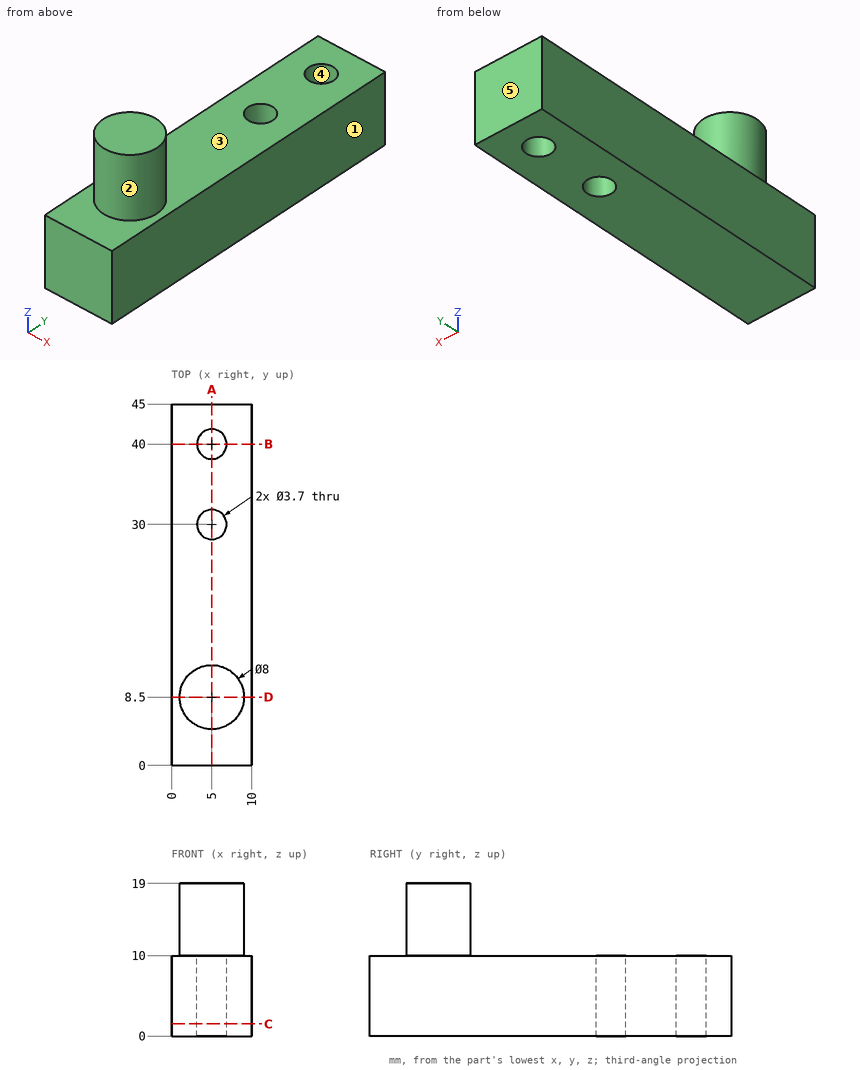
Job drawing, mm, ordinate dimensions from the low corner. One solid piece. A direction names the side the tool comes from. Give positions to 0.01 mm unless a question says otherwise; leave off trailing zeros. Loops run counter-clockwise (first coordinate to the right, second up) from the corner with the lowest first, then second, coordinate; pieces in that order, holes last. Notation, with made-up numbers: (-8, 26.25) -> (17, 26.25) arc R26 cw to (17, 40.25) -> close; hole circle Ø3 at (55.5, 30). An arc over 180 degrees is marked (long way). Use a Markdown table: item, result. Add a question column.
(1) Slice it at C-C on z = 1.5. List the corners of the cut face in (x, y).
(2) Drop a flat-ended pin along its axis: pin 1 Ø3 at (x, y) = (5.5, 24) entering from +Z. Give the stop position or say it passes through.
(3) Tool access for the marked faces 1 and 2: list every direction of +Z, -Z, +X, -X, +Y, -Y with a clear straight run to the whole face (end or side of a thin tool).
(4) Slice it at B-B on y = 40. List the corners of the cut face in (x, z), and give its area (3 significant figures).
(5) Slice it at A-A on x = 5. List the corners of the cut face in (y, z).
(6) Wall check: line 1 along Y through (x, z) = (5, 6.25); line 2 along Z through (x, y) = (9, 5.5); line 3 along X through (y, z) = (39, 8.25). Give the ranges that are in metal, low to high.
(7) Mould opens along Y. For the marked faces 3, 4 and 5 say: +Y half, -Y half, draft (parallel to the pull), parting line (faces both ways), or undercut.
(8) Slice it at D-D on y = 8.5. List the corners of the cut face in (x, z).
Filled sheet:
| question | item | result |
|---|---|---|
| 1 | outline | (0, 0) -> (10, 0) -> (10, 45) -> (0, 45) -> close; hole circle Ø3.7 at (5, 30); hole circle Ø3.7 at (5, 40) |
| 2 | pin 1 | z = 10 |
| 3 | face 1 | +Z, -Z, +X, +Y, -Y |
| 3 | face 2 | +Z |
| 4 | outline | (0, 0) -> (3.15, 0) -> (3.15, 10) -> (0, 10) -> close; (6.85, 0) -> (10, 0) -> (10, 10) -> (6.85, 10) -> close |
| 4 | area | 63.0 mm2 |
| 5 | outline | (0, 0) -> (28.15, 0) -> (28.15, 10) -> (12.5, 10) -> (12.5, 19) -> (4.5, 19) -> (4.5, 10) -> (0, 10) -> close; (31.85, 0) -> (38.15, 0) -> (38.15, 10) -> (31.85, 10) -> close; (41.85, 0) -> (45, 0) -> (45, 10) -> (41.85, 10) -> close |
| 6 | line 1 | 0 to 28.15, 31.85 to 38.15, 41.85 to 45 |
| 6 | line 2 | 0 to 10 |
| 6 | line 3 | 0 to 3.44, 6.56 to 10 |
| 7 | face 3 | draft |
| 7 | face 4 | undercut |
| 7 | face 5 | +Y half |
| 8 | outline | (0, 0) -> (10, 0) -> (10, 10) -> (9, 10) -> (9, 19) -> (1, 19) -> (1, 10) -> (0, 10) -> close |
